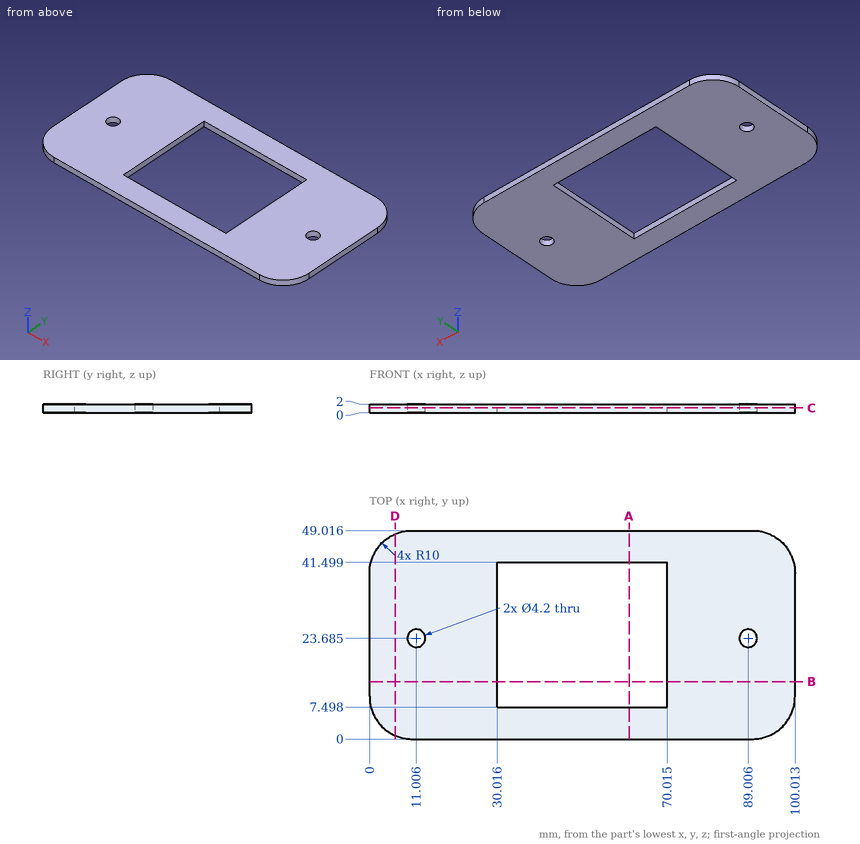
Print and shaded views of the part. All mm, measured from the part's lowest x, y and z. Give positions to 0.01 mm unless a question says otherwise; leave off trailing zeros. Order: outer loops, then holes, each group sorted by start corner. A loop starts at its lowest first (then second) coordinate and runs counter-clockwise, first axis right, second up. Notation, with made-up numbers: M 9,-18.75 L 15,-18.75 A12 ccw 15,-14.75 Z; hole C 56,56 d1. An arc over 180 degrees is marked long. Use one line per item in the form item = value.
Q1. Pin check, flat tip, straight feed: P1, Ø3.5, axis at x = 11.01, y = 23.69, coming from the -Z side. Stop position of the tip, or through.
Conclusion:
P1 = through
Q2. Slice it at C-C, the plane z = 1.1. Write the cut outline in (x, y) (1 decimal).
Conclusion:
outline = M 0,10 A10 ccw 10,0 L 90,0 A10 ccw 100,10 L 100,39 A10 ccw 90,49 L 10,49 A10 ccw 0,39 Z; hole C 11,23.7 d4.2; hole M 30,7.5 L 70,7.5 L 70,41.5 L 30,41.5 Z; hole C 89,23.7 d4.2
Q3. Wall check: probe 1 along Y at (x, z) = (67.5, 0.95) (1 decimal); probe 2 along X at (y, z) = (17, 0.7) (1 decimal); probe 3 along X at (y, z) = (24, 0.3) (1 decimal). Give the ranges that are in metal, low to high.
Conclusion:
probe_1 = 0 to 7.5, 41.5 to 49
probe_2 = 0 to 30, 70 to 100
probe_3 = 0 to 8.9, 13.1 to 30, 70 to 86.9, 91.1 to 100
Q4. Slice it at A-A, the plane x = 61. Write the cut outline in (y, z) (1 decimal).
Conclusion:
outline = M 0,0 L 7.5,0 L 7.5,2 L 0,2 Z; M 41.5,0 L 49,0 L 49,2 L 41.5,2 Z
Q5. Slice it at D-D, the plane x = 6. Write the cut outline in (y, z) (1 decimal).
Conclusion:
outline = M 0.8,0 L 48.2,0 L 48.2,2 L 0.8,2 Z
Q6. Slice it at B-B, the plane y = 13.5. Write the cut outline in (x, z) (1 decimal).
Conclusion:
outline = M 0,0 L 30,0 L 30,2 L 0,2 Z; M 70,0 L 100,0 L 100,2 L 70,2 Z
